```python
from build123d import *

# Parameters (mm, degrees)
HOLE_WIZARD_3_2_3_2_1_D = 3.2


with BuildPart() as part:
    # 草图1 → 旋转1 (revolve)
    with BuildSketch(Plane.XY):
        with BuildLine():
            Line((0, 42.25), (0, 55.25))
            Line((0, 55.25), (-5, 55.25))
            Line((-5, 55.25), (-5, 46.984704958))
            ThreePointArc((-5, 46.984704958), (-35.134118034, 31.593610905), (-47.25, 0))
            Line((-47.25, 0), (-42.25, 0))
            ThreePointArc((-42.25, 0), (-29.875261505, 29.875261505), (0, 42.25))
        make_face()
    revolve(axis=Axis((0, 0, 0), (-1, 0, 0)))

    # Ø3.2 (3.2) 直径孔1 (through all)
    with Locations(Plane(origin=(-5, 52.525, 0), x_dir=(0, 0, -1), z_dir=(-1, 0, 0))):
        with Locations((0, 0), (-45.487984334, 26.2625), (-45.487984334, 78.7875), (0, 105.05), (45.487984334, 78.7875), (45.487984334, 26.2625)):
            Hole(HOLE_WIZARD_3_2_3_2_1_D / 2)


solid = part.part
```
The model under review builds one solid part; all positions refer to its coordinate system, in mm. A direction names the side the tool comes from. Give positions to 0.01 mm unless a question says otherwise; leave off trailing zeros. Write each loop counter-clockwise with the first axis right and the second up, starting at its lowest first coordinate (ties: lowest second). Pieces come first, ordered by that corner, then holes. Notation, with made-up numbers: (-13.75, -21) - (-8.75, -21) arc R29 ccw to (-8.75, 2) - close; hole circle Ø8 at (76.25, 83.25). An arc over 180 degrees is marked (long way). Answer in a Markdown table with one row per item. Add a question column.
1. Wall thickness on line 1 along Y through (x, z) = (-1.15, 0) (3 decimals); line 2 along X through (y, z) = (47.5, 17.5); line 3 along Y through (x, z) = (-11.5, -31.5): over which ranges is each line inside the solid? List them lowest first. Write a range as [from, to].
2. We need section B-B on y = 0. Write out the cut boundary in (x, z).
3. We need section C-C on z = -13. Write out the cut boundary in (x, y), then the cut area to 3 significant figures.
4. We need section A-A on z = 0. Write out the cut boundary in (x, y) (3 decimals), then the cut area to 3 significant figures.
5. We need section D-D on x = -22. Write out the cut boundary in (y, z).
6. Insertion check: P1, Ø1.5, axis at y = 21.5, z = -24.5, coming from the +X side; P2, Ø8, axis at y = 10, z = 23, coming from the +X side; P3, Ø2, axis at x = -14, z = 1, coming from the -Y side. Each pin has a flat end and moves straight along its axis. Give the tip position at first contact, or say it passes through.
7. Draft analysis for pull direction Z (two halves, no side actions). For faces 1 (the cylindrical face through (-2.535, -11.977, 53.936)), 2 (the flat face through (0, -16, 41)), 3 (the cylindrical face through (-2.465, -53.874, 0.86)), state which applies: +Z half, -Z half, draft (parallel to the pull), parting line (faces both ways), or undercut.
8. Tool access review of faces 4 (the cylindrical face through (-2.465, -26.333, -47.086)), 5 (the flat face through (-5, 16, 45)): name each direction out of +Z, -Z, +X, -X, +Y, -Y from which nothing blocks a thin tool from reaching the whole face with its end or side.
Ans:
| question | item | result |
|---|---|---|
| 1 | line 1 | y = [-55.25, -54.125], [-50.925, -42.234], [42.234, 50.925], [54.125, 55.25] |
| 1 | line 2 | x = [-5, 0] |
| 1 | line 3 | y = [-33.29, -25.7], [25.7, 33.29] |
| 2 | outline | (-5, -55.25) - (0, -55.25) - (0, -42.25) arc R42.25 cw to (0, 42.25) - (0, 55.25) - (-5, 55.25) - (-5, 46.98) arc R47.25 ccw to (-5, -46.98) - close |
| 3 | outline | (-5, -53.7) - (0, -53.7) - (0, -40.2) arc R40.2 cw to (0, 40.2) - (0, 53.7) - (-5, 53.7) - (-5, 45.15) arc R45.43 ccw to (-5, -45.15) - close |
| 3 | area | 787 mm^2 |
| 4 | outline | (-5, -55.25) - (0, -55.25) - (0, -54.125) - (-5, -54.125) - close; (-5, -50.925) - (0, -50.925) - (0, -42.25) arc R42.25 cw to (0, 42.25) - (0, 50.925) - (-5, 50.925) - (-5, 46.985) arc R47.25 ccw to (-5, -46.985) - close; (-5, 54.125) - (0, 54.125) - (0, 55.25) - (-5, 55.25) - close |
| 4 | area | 752 mm^2 |
| 5 | outline | circle Ø83.63 at (0, 0); hole circle Ø72.14 at (0, 0) |
| 6 | P1 | stops at x = -25.94 |
| 6 | P2 | stops at x = -30.65 |
| 6 | P3 | stops at y = -45.42 |
| 7 | face 1 | parting line |
| 7 | face 2 | draft |
| 7 | face 3 | undercut |
| 8 | face 4 | +X, -X |
| 8 | face 5 | -X |
